Drawing for the job (mm, zero at the part's lowest x, y, z). A direction names the side the tool comes from. Give positions to 0.01 mm unless a question says otherwise; leave off trailing zeros. Order: outer loops, then holes, each group sorted by start corner. A loop starts at its lowest first (then second) coordinate and runs counter-clockwise, first axis right, second up. Notation, with made-up numbers: (-22.5, 46.5) - (-3.5, 46.5) arc R33 ccw to (-3.5, 82.5) - close; hole circle Ø2 at (31.25, 31). An arc over 180 degrees is marked (long way). Write each question's results on one line, items separated by ' | '. Start each with the question number.
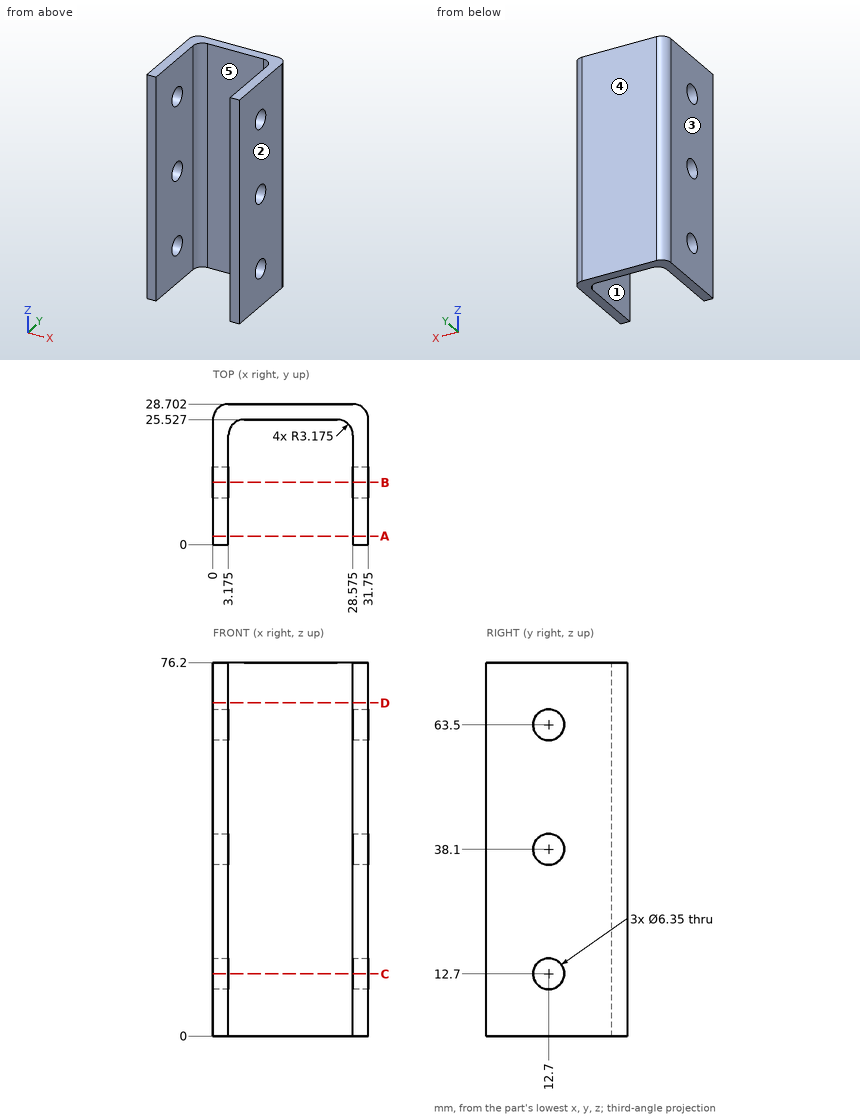
Item 1: Which spindle directions (+Z, -Z, +X, -X, +Y, -Y) get a long thin tool onto all of the face, cutting with end or side? Do the marked faces 1 and 2. Say none if no direction does.
Item 2: Cut at A-A, the plane y = 1.75. List the corners of the cut face in (x, z) (3 decimals), then the cut area to 3 significant figures.
Item 3: Two-plate mould, pull along X, no slides. Class the marked faces 3, 4 and 5: +X half, -X half, draft (parallel to the pull), parting line (faces both ways), or undercut.
Item 4: Cut at B-B, the plane y = 12.7. Count the separate pieces of the cut face and the enclosed holes in it, then the cut area to 3 significant figures.
Item 5: Probe line 1 along Z through (x, y) = (29.35, 12.7) (3 decimals); line 2 along X through (y, z) = (1.5, 63.5) (3 decimals); line 3 along Y through (x, z) = (2.35, 63.5) (3 decimals). List the from-to ranges inside material, lowest first. Write a range as from..to.
Item 6: Flat gauge pins, fed straight in: pin 1 Ø8 at (x, z) = (25, 63.5) entering from -Y; pin 2 Ø15 at (x, z) = (16.5, 55) entering from -Y. Where does each tip first touch, or does it go through?
Item 7: Cut at C-C, the plane z = 12.7. List the corners of the cut face in (x, y) (3 decimals), then the cut area to 3 significant figures.
Item 8: Cut at D-D, the plane z = 68. List the corners of the cut face in (x, y) (3 decimals).
Values found:
1) face 1: +Z, -Z, -Y | face 2: +Z, -Z, +X, +Y, -Y
2) outline: (0, 0) - (3.175, 0) - (3.175, 76.2) - (0, 76.2) - close; (28.575, 0) - (31.75, 0) - (31.75, 76.2) - (28.575, 76.2) - close | area: 484 mm2
3) face 3: -X half | face 4: draft | face 5: undercut
4) separate pieces: 8 | enclosed holes: 0 | area: 363 mm2
5) line 1: z = 0..9.525, 15.875..34.925, 41.275..60.325, 66.675..76.2 | line 2: x = 0..3.175, 28.575..31.75 | line 3: y = 0..9.525, 15.875..28.593
6) pin 1: stops at y = 0 | pin 2: stops at y = 25.53
7) outline: (0, 0) - (3.175, 0) - (3.175, 9.525) - (0, 9.525) - close; (0, 15.875) - (3.175, 15.875) - (3.175, 22.352) arc R3.175 cw to (6.35, 25.527) - (25.4, 25.527) arc R3.175 cw to (28.575, 22.352) - (28.575, 15.875) - (31.75, 15.875) - (31.75, 25.527) arc R3.175 ccw to (28.575, 28.702) - (3.175, 28.702) arc R3.175 ccw to (0, 25.527) - close; (28.575, 0) - (31.75, 0) - (31.75, 9.525) - (28.575, 9.525) - close | area: 223 mm2
8) outline: (0, 0) - (3.175, 0) - (3.175, 22.352) arc R3.175 cw to (6.35, 25.527) - (25.4, 25.527) arc R3.175 cw to (28.575, 22.352) - (28.575, 0) - (31.75, 0) - (31.75, 25.527) arc R3.175 ccw to (28.575, 28.702) - (3.175, 28.702) arc R3.175 ccw to (0, 25.527) - close
